For this review, take the finished solid that the model builds, in its own axes (mm). Face numbers are marked on the shaded views. A direction names the side the tool comes from. Give positions to 0.01 mm unless a question says otherwise; leave off trailing zeros. Order: outer loops, then holes, each group sorted by start corner. A loop starts at its lowest first (then second) coordinate and runs counter-clockwise, first axis right, second up. Notation, with made-up numbers: M 21.5,41 L 79.5,41 A9 ccw 79.5,56 Z; hole C 38.5,-17.75 d4. An arc over 180 degrees is marked long. Answer as CSV lines item,"result". Start each with the question number.
1. Machinability: for the marked faces 1, 2 and 3, which of the approach directions +Z, -Z, +X, -X, +Y, -Y give a long, thin tool a straight path to every point of the face, cutting with its end or side? Answer none if there is none.
2. Mouldability with a two-part tool opening along Z and no side actions: class the marked faces 4, 5 and 6 as pulls with the +Z half, pulls with the -Z half, needs draft (parallel to the pull), parting line crosses it, or undercut.
3. For line 1 along X through (y, z) = (25, -27.3); line 2 along X through (y, z) = (14.25, 22.2); line 3 along Z through (x, y) = (-11, 27.25), list the stretches that pass through material, from the lowest coordinate up.
4. We need section C-C, the plane y = 14.25. Give the boundary of the cut face in (x, z), and give its area (3 significant figures).
5. We need section D-D, the plane y = 4.5. Give the boundary of the cut face in (x, z).
6. We need section B-B, the plane x = -10. Give the boundary of the cut face in (y, z).
7. We need section A-A, the plane z = -27.3. Give the boundary of the cut face in (x, y).
8. Clearance check with flat-ended pins moving along their axes: P1, Ø2, axis at x = 5.5, z = 21, coming from the +Y side; P2, Ø2, axis at x = -4.5, z = 21, coming from the -Y side; P3, Ø10, axis at y = 21.5, z = -13.5, coming from the -X side; P4, Ø2.5, axis at x = -13.23, y = 20, coming from the -Z side. State where each tip first meets the part, or that it passes through.
from build123d import *

# Parameters (mm, degrees)
SKETCH2_W           = 5.98
SKETCH2_H           = 20.5
SKETCH2_R           = 1.5
SKETCH2_R_2         = 2
BOSS_EXTRUDE1_DEPTH = 28.5
SKETCH2_4_R         = 1.5
CUT_EXTRUDE1_DEPTH  = 15
SKETCH3_W           = 6.5
SKETCH3_H           = 15
BOSS_EXTRUDE2_DEPTH = 32.46
SKETCH2_5_R         = 2
CUT_EXTRUDE2_DEPTH  = 94.46
SKETCH2_6_R         = 2
CUT_EXTRUDE4_DEPTH  = 8
CUT_EXTRUDE5_START  = -8
SKETCH5_R           = 2
CUT_EXTRUDE5_DEPTH  = 8
CUT_EXTRUDE3_DEPTH  = 10
CUT_EXTRUDE6_DEPTH  = 3.5
CUT_EXTRUDE7_REACH  = 54.735
SKETCH11_W          = 41
SKETCH11_H          = 28.5
SKETCH12_R          = 1.5
CUT_EXTRUDE8_DEPTH  = 64


with BuildPart() as part:
    # Sketch2 → Boss-Extrude1 (new body)
    # profile 1 of 12: a face of its own
    with BuildSketch(Plane(origin=(0, 0, 0), x_dir=(1, 0, 0), z_dir=(0, 1, 0))):
        with Locations((-13.24, -7)):
            Rectangle(SKETCH2_W, SKETCH2_H)
        with Locations((-13.23, -13.25)):
            Circle(SKETCH2_R, mode=Mode.SUBTRACT)
    # profile 2 of 12: a face of its own
    with BuildSketch(Plane(origin=(0, 0, 0), x_dir=(1, 0, 0), z_dir=(0, 1, 0))):
        with Locations((-13.23, -13.25)):
            Circle(SKETCH2_R)
    # profile 3 of 12: a face of its own
    with BuildSketch(Plane(origin=(0, 0, 0), x_dir=(1, 0, 0), z_dir=(0, 1, 0))):
        with Locations((-13.24, 13.5)):
            Rectangle(SKETCH2_W, SKETCH2_H)
        with Locations((-13.23, 19.75)):
            Circle(SKETCH2_R, mode=Mode.SUBTRACT)
    # profile 4 of 12: a face of its own
    with BuildSketch(Plane(origin=(0, 0, 0), x_dir=(1, 0, 0), z_dir=(0, 1, 0))):
        with Locations((-13.23, 19.75)):
            Circle(SKETCH2_R)
    # profile 5 of 12: a face of its own
    with BuildSketch(Plane(origin=(0, 0, 0), x_dir=(1, 0, 0), z_dir=(0, 1, 0))):
        with Locations((13.24, 13.5)):
            Rectangle(SKETCH2_W, SKETCH2_H)
        with Locations((13.23, 19.75)):
            Circle(SKETCH2_R, mode=Mode.SUBTRACT)
    # profile 6 of 12: a face of its own
    with BuildSketch(Plane(origin=(0, 0, 0), x_dir=(1, 0, 0), z_dir=(0, 1, 0))):
        with Locations((13.23, 19.75)):
            Circle(SKETCH2_R)
    # profile 7 of 12: a face of its own
    with BuildSketch(Plane(origin=(0, 0, 0), x_dir=(1, 0, 0), z_dir=(0, 1, 0))):
        with Locations((13.24, -7)):
            Rectangle(SKETCH2_W, SKETCH2_H)
        with Locations((13.23, -13.25)):
            Circle(SKETCH2_R, mode=Mode.SUBTRACT)
    # profile 8 of 12: a face of its own
    with BuildSketch(Plane(origin=(0, 0, 0), x_dir=(1, 0, 0), z_dir=(0, 1, 0))):
        with Locations((13.23, -13.25)):
            Circle(SKETCH2_R)
    # profile 9 of 12: a face of its own
    with BuildSketch(Plane(origin=(0, 0, 0), x_dir=(1, 0, 0), z_dir=(0, 1, 0))):
        Polygon((0, -23.75), (0, -17.25), (-10.25, -17.25), (-16.23, -17.25), (-16.23, -23.75), align=None)
        with Locations((-4.95, -20.8)):
            Circle(SKETCH2_R_2, mode=Mode.SUBTRACT)
    # profile 10 of 12: a face of its own
    with BuildSketch(Plane(origin=(0, 0, 0), x_dir=(1, 0, 0), z_dir=(0, 1, 0))):
        with Locations((-4.95, -20.8)):
            Circle(SKETCH2_R_2)
    # profile 11 of 12: a face of its own
    with BuildSketch(Plane(origin=(0, 0, 0), x_dir=(1, 0, 0), z_dir=(0, 1, 0))):
        Polygon((10.25, -17.25), (0, -17.25), (0, -23.75), (16.23, -23.75), (16.23, -17.25), align=None)
        with Locations((4.95, -20.8)):
            Circle(SKETCH2_R_2, mode=Mode.SUBTRACT)
    # profile 12 of 12: a face of its own
    with BuildSketch(Plane(origin=(0, 0, 0), x_dir=(1, 0, 0), z_dir=(0, 1, 0))):
        with Locations((4.95, -20.8)):
            Circle(SKETCH2_R_2)
    extrude(amount=BOSS_EXTRUDE1_DEPTH)

    # Sketch2_4 → Cut-Extrude1 (cut)
    with BuildSketch(Plane(origin=(0, 0, 0), x_dir=(1, 0, 0), z_dir=(0, 1, 0))):
        with Locations(Location((13.23, 19.75, 0), (0, 0, 270))):
            Circle(SKETCH2_4_R)
        with Locations(Location((-13.23, 19.75, 0), (0, 0, 270))):
            Circle(SKETCH2_4_R)
        with Locations(Location((-13.23, -13.25, 0), (0, 0, 270))):
            Circle(SKETCH2_4_R)
        with Locations(Location((13.23, -13.25, 0), (0, 0, 270))):
            Circle(SKETCH2_4_R)
    extrude(amount=CUT_EXTRUDE1_DEPTH, mode=Mode.SUBTRACT)

    # Sketch3 → Boss-Extrude2 (add)
    with BuildSketch(Plane.ZY.offset(16.23)):
        with Locations((-27, 21)):
            Rectangle(SKETCH3_W, SKETCH3_H)
    extrude(amount=-BOSS_EXTRUDE2_DEPTH)

    # Sketch2_5 → Cut-Extrude2 (cut)
    with BuildSketch(Plane(origin=(0, 0, 0), x_dir=(1, 0, 0), z_dir=(0, 1, 0))):
        with Locations(Location((-4.95, 27.3, 0), (0, 0, 90))):
            Circle(SKETCH2_5_R)
        with Locations(Location((4.95, 27.3, 0), (0, 0, 90))):
            Circle(SKETCH2_5_R)
    extrude(amount=CUT_EXTRUDE2_DEPTH, mode=Mode.SUBTRACT)

    # Sketch2_6 → Cut-Extrude4 (cut)
    with BuildSketch(Plane(origin=(0, 0, 0), x_dir=(1, 0, 0), z_dir=(0, 1, 0))):
        with Locations(Location((-4.95, -20.8, 0), (0, 0, 270))):
            Circle(SKETCH2_6_R)
        with Locations(Location((4.95, -20.8, 0), (0, 0, 270))):
            Circle(SKETCH2_6_R)
    extrude(amount=CUT_EXTRUDE4_DEPTH, mode=Mode.SUBTRACT)

    # Sketch5 → Cut-Extrude5 (cut)
    with BuildSketch(Plane(origin=(0, 28.5, 0), x_dir=(1, 0, 0), z_dir=(0, 1, 0)).offset(CUT_EXTRUDE5_START)):
        with Locations(Location((-4.95, -20.8, 0), (0, 0, 270))):
            Circle(SKETCH5_R)
        with Locations(Location((4.95, -20.8, 0), (0, 0, 270))):
            Circle(SKETCH5_R)
    extrude(amount=CUT_EXTRUDE5_DEPTH, mode=Mode.SUBTRACT)

    # Sketch4 → Cut-Extrude3 (cut)
    with BuildSketch(Plane(origin=(0, 0, 17.25), x_dir=(-1, 0, 0), z_dir=(0, 0, -1))):
        with BuildLine():
            ThreePointArc((-3.5, 14.25), (-5, 15.75), (-6.5, 14.25))
            Line((-6.5, 14.25), (-3.5, 14.25))
        make_face()
        with BuildLine():
            Line((-3.5, 14.25), (-6.5, 14.25))
            ThreePointArc((-6.5, 14.25), (-5, 12.75), (-3.5, 14.25))
        make_face()
        with BuildLine():
            ThreePointArc((6.5, 14.25), (5, 15.75), (3.5, 14.25))
            Line((3.5, 14.25), (6.5, 14.25))
        make_face()
        with BuildLine():
            Line((6.5, 14.25), (3.5, 14.25))
            ThreePointArc((3.5, 14.25), (5, 12.75), (6.5, 14.25))
        make_face()
    extrude(amount=-CUT_EXTRUDE3_DEPTH, mode=Mode.SUBTRACT)

    # Sketch4_3 → Cut-Extrude6 (cut)
    with BuildSketch(Plane(origin=(0, 0, 17.25), x_dir=(-1, 0, 0), z_dir=(0, 0, -1))):
        with BuildLine():
            ThreePointArc((-2, 14.25), (-5, 17.25), (-8, 14.25))
            Line((-8, 14.25), (-6.5, 14.25))
            ThreePointArc((-6.5, 14.25), (-5, 15.75), (-3.5, 14.25))
            Line((-3.5, 14.25), (-2, 14.25))
        make_face()
        with BuildLine():
            Line((-6.5, 14.25), (-8, 14.25))
            ThreePointArc((-8, 14.25), (-5, 11.25), (-2, 14.25))
            Line((-2, 14.25), (-3.5, 14.25))
            ThreePointArc((-3.5, 14.25), (-5, 12.75), (-6.5, 14.25))
        make_face()
        with BuildLine():
            ThreePointArc((8, 14.25), (5, 17.25), (2, 14.25))
            Line((2, 14.25), (3.5, 14.25))
            ThreePointArc((3.5, 14.25), (5, 15.75), (6.5, 14.25))
            Line((6.5, 14.25), (8, 14.25))
        make_face()
        with BuildLine():
            Line((3.5, 14.25), (2, 14.25))
            ThreePointArc((2, 14.25), (5, 11.25), (8, 14.25))
            Line((8, 14.25), (6.5, 14.25))
            ThreePointArc((6.5, 14.25), (5, 12.75), (3.5, 14.25))
        make_face()
    extrude(amount=-CUT_EXTRUDE6_DEPTH, mode=Mode.SUBTRACT)

    # Sketch11 → Cut-Extrude7 (cut, up to next)
    with BuildSketch(Plane.ZY.offset(16.23), mode=Mode.PRIVATE) as cut_extrude7_sk1:
        with Locations((-3.25, 14.25)):
            Rectangle(SKETCH11_W, SKETCH11_H)
    cut_extrude7_tool1 = extrude(cut_extrude7_sk1.sketch, amount=-CUT_EXTRUDE7_REACH, mode=Mode.PRIVATE) & part.part
    add(cut_extrude7_tool1.solids().sort_by_distance((-16.23, 14.25, -3.25))[0], mode=Mode.SUBTRACT)

    # Sketch12 → Cut-Extrude8 (cut)
    with BuildSketch(Plane(origin=(0, 0, -30.25), x_dir=(-1, 0, 0), z_dir=(0, 0, -1))):
        with Locations(Location((13.23, 20, 0), (0, 0, 90))):
            Circle(SKETCH12_R)
        with Locations(Location((13.23, 8, 0), (0, 0, 90))):
            Circle(SKETCH12_R)
    extrude(amount=-CUT_EXTRUDE8_DEPTH, mode=Mode.SUBTRACT)


solid = part.part
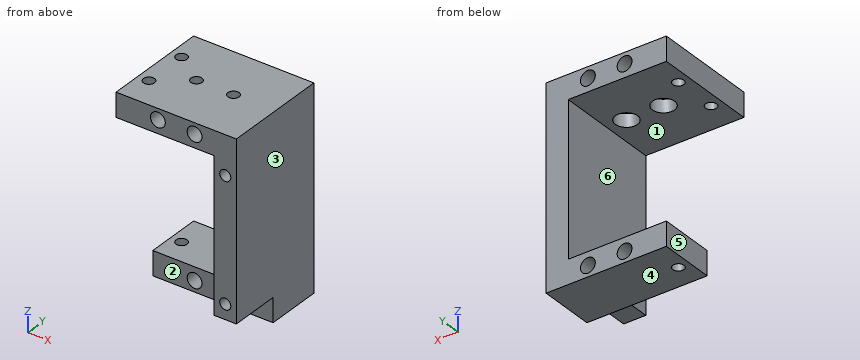
Result set:
1,face 1,"-X, +Y, -Y"
1,face 2,"-Z, +X, -X, -Y"
1,face 3,"+Z, -Z, +X, +Y, -Y"
2,face 4,"pulls with the -Z half"
2,face 5,"needs draft"
2,face 6,"undercut"
3,line 1,"-16.23 to -6.95, -2.95 to 2.95, 6.95 to 16.23"
3,line 2,"-16.23 to -6.5, -3.5 to 3.5, 6.5 to 16.23"
3,line 3,"-30.25 to -23.75, 17.25 to 23.75"
4,outline,"M -16.23,-30.25 L 16.23,-30.25 L 16.23,23.75 L 6.5,23.75 L 6.5,20.75 L 8,20.75 L 8,17.25 L 10.25,17.25 L 10.25,-23.75 L -16.23,-23.75 Z; M -16.23,17.25 L -8,17.25 L -8,20.75 L -6.5,20.75 L -6.5,23.75 L -16.23,23.75 Z; M -3.5,20.75 L -2,20.75 L -2,17.25 L 2,17.25 L 2,20.75 L 3.5,20.75 L 3.5,23.75 L -3.5,23.75 Z; hole C -4.95,-27.3 d4; hole C 4.95,-27.3 d4; hole C 13.23,-19.75 d3; hole C 13.23,13.25 d3"
4,area,"568 mm2"
5,outline,"M -16.23,17.25 L 10.25,17.25 L 10.25,-23.75 L 16.23,-23.75 L 16.23,23.75 L -16.23,23.75 Z; hole C -4.95,20.8 d4; hole C 4.95,20.8 d4; hole C 13.23,-19.75 d3; hole C 13.23,13.25 d3"
6,outline,"M 0,17.25 L 28.5,17.25 L 28.5,23.75 L 0,23.75 Z; M 13.5,-30.25 L 28.5,-30.25 L 28.5,-23.75 L 13.5,-23.75 Z"
7,outline,"M -16.23,13.5 L -6.95,13.5 L -6.95,28.5 L -16.23,28.5 Z; M -2.95,13.5 L 2.95,13.5 L 2.95,28.5 L -2.95,28.5 Z; M 6.95,13.5 L 16.23,13.5 L 16.23,28.5 L 6.95,28.5 Z; hole C -13.23,20 d3"
8,P1,"y = 20.5"
8,P2,"y = 8"
8,P3,"x = 10.25"
8,P4,"through"
